```python
from build123d import *

# Parameters (mm, degrees)
F0_R        = 19.417133546
F0_W        = 2.5
F0_H        = 26
F1_DEPTH    = 5
F2_SIZE     = 4.99999
F3_DEPTH    = 40
F3_FACE_W   = 6.5
F3_FACE_H   = 30
F3_FACE_W_2 = 2.5
F3_FACE_H_2 = 26
F4_ANGLE    = 15
F6_DEPTH    = 40
F7_W        = 0.5
F7_H        = 16
F8_DEPTH    = 25
F9_DEPTH    = 15


# Not quite as in the source:
# - a fillet or chamfer is up to 0.001 mm smaller than in the source, because OpenCascade refuses the exact size


with BuildPart() as f1:
    # F0 (on Front) → F1 (new body)
    with BuildSketch(Plane.XZ):
        Circle(F0_R)
        with BuildLine():
            ThreePointArc((3.25, 13.6175438314), (10.9886304879, 8.6746757864), (14, 0))
            ThreePointArc((14, 0), (10.9886304879, -8.6746757864), (3.25, -13.6175438314))
            Line((3.25, -13.6175438314), (3.25, -15))
            Line((3.25, -15), (-3.25, -15))
            Line((-3.25, -15), (-3.25, -13.6175438314))
            ThreePointArc((-3.25, -13.6175438314), (-14, 0), (-3.25, 13.6175438314))
            Line((-3.25, 13.6175438314), (-3.25, 15))
            Line((-3.25, 15), (3.25, 15))
            Line((3.25, 15), (3.25, 13.6175438314))
        make_face(mode=Mode.SUBTRACT)
        with BuildLine():
            Line((-3.25, -13.6175438314), (-3.25, 13.6175438314))
            ThreePointArc((-3.25, 13.6175438314), (-14, 0), (-3.25, -13.6175438314))
        make_face()
        with BuildLine():
            ThreePointArc((3.25, -13.6175438314), (10.9886304879, -8.6746757864), (14, 0))
            ThreePointArc((14, 0), (10.9886304879, 8.6746757864), (3.25, 13.6175438314))
            Line((3.25, 13.6175438314), (3.25, -13.6175438314))
        make_face()
        with BuildLine():
            Line((3.25, -13.6175438314), (3.25, 13.6175438314))
            ThreePointArc((3.25, 13.6175438314), (0, 14), (-3.25, 13.6175438314))
            Line((-3.25, 13.6175438314), (-3.25, -13.6175438314))
            ThreePointArc((-3.25, -13.6175438314), (0, -14), (3.25, -13.6175438314))
        make_face()
        Rectangle(F0_W, F0_H, mode=Mode.SUBTRACT)
        with BuildLine():
            Line((3.25, -15), (3.25, -13.6175438314))
            ThreePointArc((3.25, -13.6175438314), (0, -14), (-3.25, -13.6175438314))
            Line((-3.25, -13.6175438314), (-3.25, -15))
            Line((-3.25, -15), (3.25, -15))
        make_face()
        with BuildLine():
            ThreePointArc((-3.25, 13.6175438314), (0, 14), (3.25, 13.6175438314))
            Line((3.25, 13.6175438314), (3.25, 15))
            Line((3.25, 15), (-3.25, 15))
            Line((-3.25, 15), (-3.25, 13.6175438314))
        make_face()
    extrude(amount=F1_DEPTH)

    # F2 (size 5 in the source; OpenCascade refuses exactly that, so slightly less here)
    f2_edges = [f1.edges().sort_by_distance(p)[0] for p in [
        (-19.417134, -5, 0),
    ]]
    chamfer(f2_edges, length=F2_SIZE)

    # F0 (on Front) → F3 (join)
    with BuildSketch(Plane.XZ):
        with BuildLine():
            ThreePointArc((-3.25, 13.6175438314), (0, 14), (3.25, 13.6175438314))
            Line((3.25, 13.6175438314), (3.25, 15))
            Line((3.25, 15), (-3.25, 15))
            Line((-3.25, 15), (-3.25, 13.6175438314))
        make_face()
        with BuildLine():
            Line((3.25, -13.6175438314), (3.25, 13.6175438314))
            ThreePointArc((3.25, 13.6175438314), (0, 14), (-3.25, 13.6175438314))
            Line((-3.25, 13.6175438314), (-3.25, -13.6175438314))
            ThreePointArc((-3.25, -13.6175438314), (0, -14), (3.25, -13.6175438314))
        make_face()
        Rectangle(F0_W, F0_H, mode=Mode.SUBTRACT)
        with BuildLine():
            Line((3.25, -15), (3.25, -13.6175438314))
            ThreePointArc((3.25, -13.6175438314), (0, -14), (-3.25, -13.6175438314))
            Line((-3.25, -13.6175438314), (-3.25, -15))
            Line((-3.25, -15), (3.25, -15))
        make_face()
    extrude(amount=-F3_DEPTH)

    # F3_face (on face) → F4 (revolve)
    with BuildSketch(Plane(origin=(0, 40, 0), x_dir=(1, 0, 0), z_dir=(0, 1, 0))):
        Rectangle(F3_FACE_W, F3_FACE_H)
        Rectangle(F3_FACE_W_2, F3_FACE_H_2, mode=Mode.SUBTRACT)
    revolve(axis=Axis((0, 40, -15), (-1, 0, 0)), revolution_arc=F4_ANGLE)

    # F5 (on face) → F6 (join)
    with BuildSketch(Plane(origin=(0, 41.0705080757, -11.0048094716), x_dir=(-1, 0, 0), z_dir=(0, 0.9659258263, -0.2588190451))):
        Polygon((3.25, -4.1361255902), (3.25, 11.1839016899), (1.25, 11.1839016899), (1.25, -2.1361255902), (-1.25, -2.1361255902), (-1.25, 11.1839016899), (-3.25, 11.1839016899), (-3.25, -4.1361255902), align=None)
    extrude(amount=F6_DEPTH)

    # F7 (on face) → F8 (cut)
    with BuildSketch(Plane(origin=(-3.25, 0, 0), x_dir=(0, -1, 0), z_dir=(-1, 0, 0))):
        with Locations((-32.7866710722, 0)):
            Rectangle(F7_W, F7_H)
    extrude(amount=-F8_DEPTH, mode=Mode.SUBTRACT)

    # F0 (on Front) → F9 (join)
    with BuildSketch(Plane.XZ):
        with BuildLine():
            ThreePointArc((3.25, -13.6175438314), (10.9886304879, -8.6746757864), (14, 0))
            ThreePointArc((14, 0), (10.9886304879, 8.6746757864), (3.25, 13.6175438314))
            Line((3.25, 13.6175438314), (3.25, -13.6175438314))
        make_face()
        with BuildLine():
            Line((-3.25, -13.6175438314), (-3.25, 13.6175438314))
            ThreePointArc((-3.25, 13.6175438314), (-14, 0), (-3.25, -13.6175438314))
        make_face()
    extrude(amount=-F9_DEPTH)


solid = f1.part
```
Geometry check sheet. Reference: the model listing, model coordinates, mm. A direction names the side the tool comes from. Give positions to 0.01 mm unless a question says otherwise; leave off trailing zeros. Write each loop counter-clockwise with the first axis right and the second up, starting at its lowest first coordinate (ties: lowest second). Pieces come first, ordered by that corner, then holes. Notation, with made-up numbers: (1, -3) - (28, -3) arc R24 ccw to (28, 23) - close; hole circle Ø8 at (-37.5, -32). An arc over 180 degrees is marked (long way). Use a Markdown table: item, result.
Q1. Set-up check for faces 4 (the face through (-14, 7, 0)), 5 (the face through (0, 20, -15)), 6 (the face through (-8, 15, 0)), 7 (the face through (-0.017, 59.566, -18.172)), 8 (the face through (-2, 32.537, 0)): record each of +Z, -Z, +X, -X, +Y, -Y from which the full face is reachable in a straight line by a thin tool's end or side.
Computed:
| item | result |
|---|---|
| face 4 | -X, +Y |
| face 5 | -Z, +X, -X |
| face 6 | +Z, -Z, -X, +Y |
| face 7 | +Y |
| face 8 | +X, -X |
Q2. Section check B-B, the plane y = 51. Enter the section's corners in (x, z), then the cut area to 3 significant figures.
Computed:
| item | result |
|---|---|
| outline | (-3.25, -17.95) - (3.25, -17.95) - (3.25, -2.09) - (1.25, -2.09) - (1.25, -15.88) - (-1.25, -15.88) - (-1.25, -2.09) - (-3.25, -2.09) - close |
| area | 68.6 mm² |
Q3. Go/stop test with flat-tipped pins: P1, Ø12, axis at x = -11, z = -5, coming from the +Y side; P2, Ø12, axis at y = 50, z = -4, coming from the -X side; P3, Ø4, axis at x = -13, z = -11, coming from the -Y side; P4, Ø1, axis at x = -14, z = -4.5, coming from the -Y side. Record where each tip stops, or that it passes through.
Computed:
| item | result |
|---|---|
| P1 | stops at y = 15 |
| P2 | stops at x = -3.25 |
| P3 | stops at y = -4.39 |
| P4 | stops at y = -5 |
Q4. Thickness scan on L1, parallel to X at y = 29, z = 0; L2, parallel to Y at x = -8.5, z = -7.5; L3, parallel to X at y = 4.5, z = 7. Record the ranges inside material, lowest first. Write a range as [from, to].
Computed:
| item | result |
|---|---|
| L1 | x = [-3.25, -1.25], [1.25, 3.25] |
| L2 | y = [-5, 15] |
| L3 | x = [-12.12, -1.25], [1.25, 12.12] |
Q5. Draft check along Z on faces 1 (the face through (0, 17, -13)), 2 (the face through (3.25, 39, -4)), 3 (the face through (0, 20, 15)). Enter one of: pulls with the +Z half, pulls with the -Z half, needs draft (parallel to the pull), parting line crosses it, or undercut.
Computed:
| item | result |
|---|---|
| face 1 | undercut |
| face 2 | needs draft |
| face 3 | pulls with the +Z half |
Q6. Section check C-C, the plane z = -6. Give the number of separate pieces and of enclosed holes in the cut face, then the cut area to 3 significant figures.
Computed:
| item | result |
|---|---|
| separate pieces | 4 |
| enclosed holes | 0 |
| area | 688 mm² |
